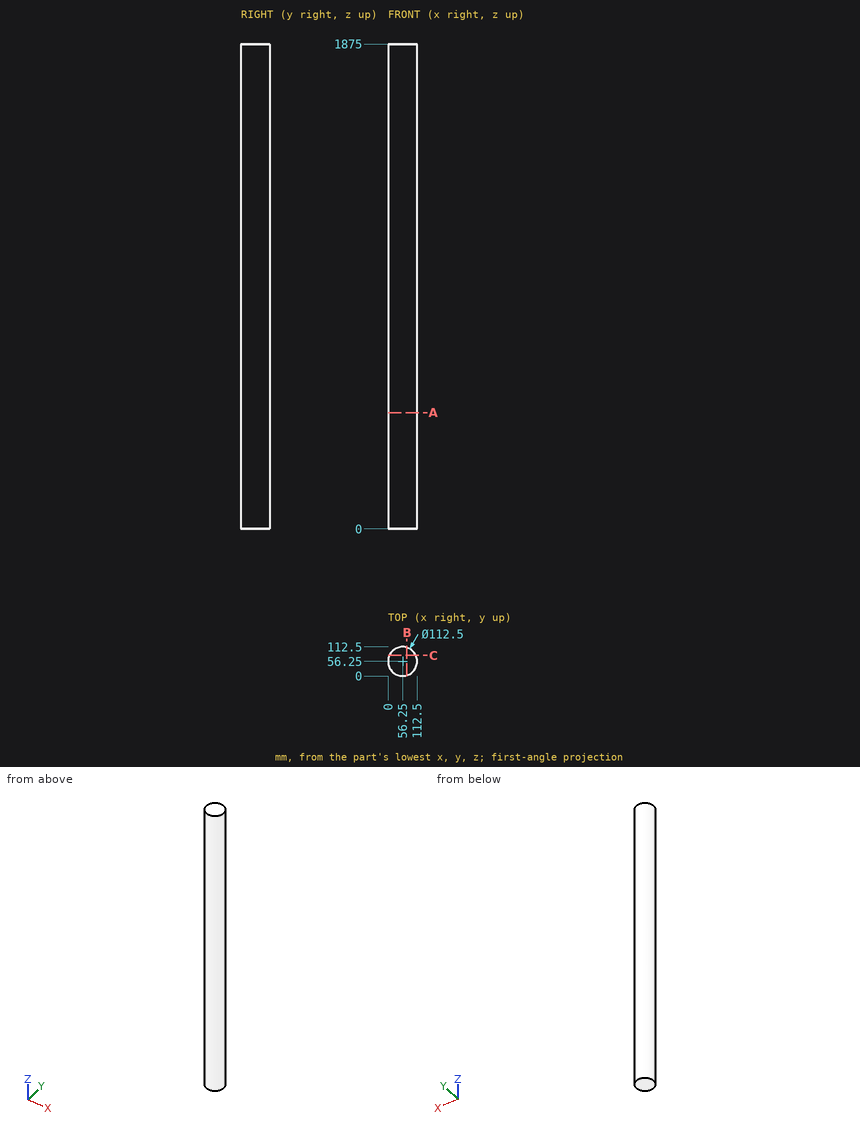
Job drawing, mm, ordinate dimensions from the low corner. One solid piece. Round coordinates to 2 decimals unless told otherwise and drop trailing zeros. Loops run counter-clockwise (first coordinate to the right, second up) from the corner with the lowest first, then second, coordinate; pieces in that order, holes last. Notation, with made-up numbers: (41, 79.5) -> (86, 79.5) arc R20 cw to (86, 91.5) -> close; hole circle Ø7 at (39, -40). An arc over 180 degrees is marked (long way). Use CSV: the item, a comma, the result in double quotes. Start each with the question number.
Q1. Drill centre lines: L1, parallel to Y at x = 51.5, z = 1421.5; L2, parallel to X at y = 57.5, z = 592. Where is each one in solid material? Low to high.
Q2. Saw through at B-B on x = 73. Give the cut face in (y, z).
Q3. Saw through at A-A on z = 449.5. Give the cut face in (x, y), and give its area (3 significant figures).
Q4. Saw through at C-C on y = 80. Give the cut face in (x, z), and give its area (3 significant figures).
Q5. Flat gauge pins, fed straight in: pin 1 Ø10 at (y, z) = (47, 1226.5) entering from +X; pin 2 Ø10 at (y, z) = (66, 400) entering from -X; pin 3 Ø3 at (x, z) = (75.5, 1224.5) entering from -Y. Where does each tip first touch, or does it go through?
Solutions:
1,L1,"y = 0.2 to 112.3"
1,L2,"x = 0.01 to 112.49"
2,outline,"(2.55, 0) -> (109.95, 0) -> (109.95, 1875) -> (2.55, 1875) -> close"
3,outline,"circle Ø112.5 at (56.25, 56.25)"
3,area,"9,940 mm^2"
4,outline,"(5.26, 0) -> (107.24, 0) -> (107.24, 1875) -> (5.26, 1875) -> close"
4,area,"191,000 mm^2"
5,pin 1,"stops at x = 112.34"
5,pin 2,"stops at x = 0.2"
5,pin 3,"stops at y = 2.87"
